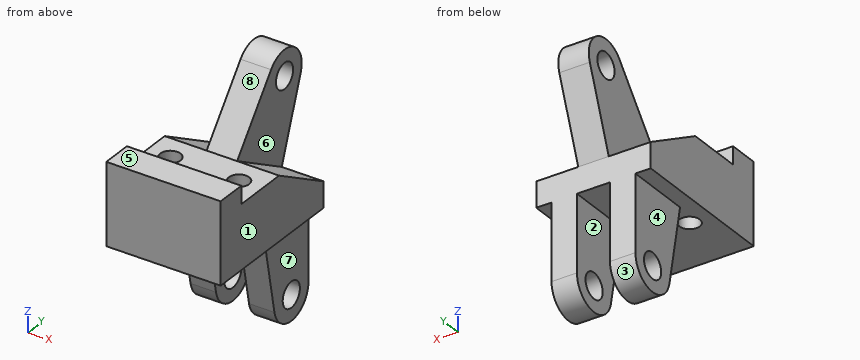
Autodesk Inventor part; units mm, degrees
ref_plane "YZ Plane" through (0, 0, 0) normal (1, 0, 0) x (0, 1, 0)
ref_plane "XZ Plane" through (0, 0, 0) normal (0, 1, 0) x (-1, 0, 0)
ref_plane "XY Plane" through (0, 0, 0) normal (0, 0, 1) x (1, 0, 0)
sketch "Szkic1" plane through (0, 0, 0) normal (0, 1, 0) x (-1, 0, 0)
  line L0 (0, 0) -> (-45, 0)
  line L1 (-45, 0) -> (-45, 32)
  line L2 (-45, 32) -> (0, 32)
  line L3 (0, 32) -> (0, 0)
  dimension "d0" = 45
  dimension "d1" = 32
extrude "Wyciągnięcie proste1" add sketch "Szkic1" along normal blind 12
sketch "Szkic2" plane through (0, 12, 0) normal (0, 1, 0) x (1, 0, 0)
  line L0 (45, 0) -> (0, 0)
  line L1 (45, -32) -> (45, 0)
  line L2 (0, 0) -> (45, 0)
  line L3 (45, 0) -> (45, -25)
  line L4 (45, -25) -> (0, -25)
  line L5 (0, -25) -> (0, 0)
extrude "Wyciągnięcie proste2" add sketch "Szkic2" along normal blind 48
sketch "Szkic3" plane through (0, 12, 25) normal (0, 0, 1) x (1, 0, 0)
  point P0 (0, -12)
  point P1 (9, 12)
  point P2 (36, 12)
hole "Otwór1" at (9, 24, 25) at (36, 24, 25) direction (0, 0, -1) diameter 8 end through all
chamfer "Faza1" distance 26 angle 30 1 edges at (22.5, 60, 25) measured on face at (26.3804, 49.1806, 25)
sketch "Szkic4" plane through (0, 60, 0) normal (0, 1, 0) x (1, 0, 0)
  point P0 (0, 0)
ref_plane "Płaszczyzna konstrukcyjna1" through (22.5, 0, 32) normal (1, 0, 0) x (0, 0, -1)
sketch "Szkic5" plane through (22.5, 0, 32) normal (1, 0, 0) x (0, 0, -1)
  circle A0 centre (-11.7045, 61.6029) radius 10
  line L0 (7, 34) -> (22.0111, 60)
  line L1 (22.0111, 60) -> (-8.2916, 71.0025)
  line L2 (7, 12) -> (7, 34)
  line L3 (7, 34) -> (-17.9194, 53.7687)
  point P0 (32, 0)
  dimension "d16" = 20
  dimension "d17" = 30
extrude "Wyciągnięcie proste3" add sketch "Szkic5" along normal mid plane 12
sketch "Szkic6" plane through (28.5, 0, 32) normal (1, 0, 0) x (0, 0, -1)
  arc A0 (-8.2916, 71.0025) -> (-17.9194, 53.7687) centre (-11.7045, 61.6029) ccw
  point P0 (32, 0)
hole "Otwór2" at (28.5, 61.6029, 43.7045) direction (-1, 0, 0) diameter 10 end through all
sketch "Szkic7" plane through (28.5, 0, 32) normal (1, 0, 0) x (0, 0, -1)
  point P0 (32, 0)
sketch "Szkic8" plane through (22.5, 0, 32) normal (1, 0, 0) x (0, 0, -1)
  circle A0 centre (62, 50) radius 10
  line L0 (32, 0) -> (32, 60)
  line L1 (32, 60) -> (62, 60)
  line L2 (32, 34) -> (63.9026, 40.1827)
  dimension "d27" = 20
  dimension "d28" = 30
  dimension "d30" = 26
extrude "Wyciągnięcie proste4" add sketch "Szkic8" along normal mid plane 33
sketch "Szkic9" plane through (22.5, 0, 32) normal (1, 0, 0) x (0, 0, -1)
  arc A0 (63.9026, 40.1827) -> (62, 60) centre (62, 50) ccw
  line L0 (32, 60) -> (22.0111, 60)
  line L1 (62, 60) -> (32, 60)
  line L2 (32, 60) -> (32, 34)
  line L3 (32, 0) -> (32, 60)
  line L4 (32, 34) -> (63.9026, 40.1827)
  line L5 (62, 60) -> (32, 60)
  arc A1 (63.9026, 40.1827) -> (62, 60) centre (62.5165, 50.0496) ccw
extrude "Wyciągnięcie proste5" cut sketch "Szkic9" along normal mid plane 13 contours L4 L2 L1 A0
sketch "Szkic10" plane through (39, 0, 32) normal (1, 0, 0) x (0, 0, -1)
  point P0 (32, 0)
sketch "Szkic11" plane through (39, 0, 32) normal (1, 0, 0) x (0, 0, -1)
  arc A0 (63.9026, 40.1827) -> (62, 60) centre (62, 50) ccw
  point P0 (32, 0)
hole "Otwór3" at (39, 50, -30) direction (-1, 0, 0) diameter 10 end through all
Could you check a few things on this model? Use its own coordinates, in mm. Face numbers are marked on the shaded views. A direction names the side the tool comes from. Coordinates: 2 decimals unless noted, no trailing zeros. Loops run counter-clockwise (first coordinate to the right, second up) from the corner with the lowest first, then second, coordinate; pieces in that order, holes last.
1. Imagine slicing it at D-D (z = 12). Please give me the cut outline in (x, y).
2. For P1, Ø1.5, axis at x = 15.5, y = 21, coming from the +Z side; P2, Ø11.5, axis at y = 45, z = 35.5, coming from the +X side; P3, Ø8, axis at y = 53, z = -14, coming from the -X side, each with a flat end and sliding along its axis, tell me the tip position at first contact or that it passes through.
3. Imagine slicing it at C-C (z = -9). Please give me the cut outline in (x, y).
4. For the marked faces 4, 5, 6, 7 and 8, which set-ups out of +Z, -Z, +X, -X, +Y, -Y let a thin tool reach every point of the face, with its end or its side?
5. Imagine slicing it at A-A (x = 9). Please give me the cut outline in (y, z).
6. I need wall thicknesses on L1, parallel to X at y = 24, z = 18; L2, parallel to Y at x = 9, z = 16.5; L3, parallel to Y at x = 9, z = 5. Which ranges of each line are inside material? Lowest first, please.
7. Imagine slicing it at B-B (y = 24). Please give me the cut outline in (x, z).
8. We'd pull the mould along X, two halves only. Please class the marked faces 1, 2 and 3: released by +X, released by -X, zero draft, split by the parting line, or undercut.
Computed values:
1. outline: (0, 0) - (45, 0) - (45, 56.52) - (28.5, 56.52) - (28.5, 60.73) - (16.5, 60.73) - (16.5, 56.52) - (0, 56.52) - close; hole circle Ø8 at (9, 24); hole circle Ø8 at (36, 24)
2. P1: stops at z = 25
2. P2: stops at x = 28.5
2. P3: stops at x = 6
3. outline: (6, 35.74) - (16, 35.74) - (16, 60) - (6, 60) - close; (29, 35.74) - (39, 35.74) - (39, 60) - (29, 60) - close
4. face 4: -Z, -X, +Y, -Y
4. face 5: +Z, +X, -X, -Y
4. face 6: +Z, +X, +Y
4. face 7: -Z, +X, +Y, -Y
4. face 8: +Z, +X, -X
5. outline: (0, 0) - (20, 0) - (20, 25) - (12, 25) - (12, 32) - (0, 32) - close; (28, 0) - (34, 0) - (40.18, -31.9) arc R10 ccw to (60, -30) - (60, 9.99) - (34, 25) - (28, 25) - close; hole circle Ø10 at (50, -30)
6. L1: x = 0 to 5, 13 to 32, 40 to 45
6. L2: y = 0 to 20, 28 to 48.72
6. L3: y = 0 to 20, 28 to 60
7. outline: (0, 0) - (5, 0) - (5, 25) - (0, 25) - close; (13, 0) - (32, 0) - (32, 25) - (13, 25) - close; (40, 0) - (45, 0) - (45, 25) - (40, 25) - close
8. face 1: released by +X
8. face 2: undercut
8. face 3: zero draft
